from build123d import *

# Parameters (mm, degrees)
SKETCH1_W                    = 45.4
SKETCH1_H                    = 27
BOSS_EXTRUDE1_DEPTH          = 6
SKETCH4_W                    = 45.4
SKETCH4_H                    = 6
BOSS_EXTRUDE2_DEPTH          = 35
FILLET3_R                    = 10
F_3_0MM_DOWEL_HOLE1_D        = 3
BOSS_EXTRUDE3_DEPTH          = 6
FILLET4_R                    = 6
F_3_0_3_DIAMETER_HOLE1_D     = 3
F_3_0_3_DIAMETER_HOLE1_DEPTH = 6
F_3_0_3_DIAMETER_HOLE1_TIP   = 0.901290929
F_3_0_3_DIAMETER_HOLE2_D     = 3
F_3_0_3_DIAMETER_HOLE2_DEPTH = 6
F_3_0_3_DIAMETER_HOLE2_TIP   = 0.901290929


with BuildPart() as part:
    # Sketch1 → Boss-Extrude1 (new body)
    with BuildSketch(Plane(origin=(0, 0, 0), x_dir=(1, 0, 0), z_dir=(0, 1, 0))):
        with Locations((22.7, 13.5)):
            Rectangle(SKETCH1_W, SKETCH1_H)
    extrude(amount=BOSS_EXTRUDE1_DEPTH)

    # Sketch4 → Boss-Extrude2 (add)
    with BuildSketch(Plane(origin=(0, 6, 0), x_dir=(1, 0, 0), z_dir=(0, 1, 0))):
        with Locations((22.7, 13.5)):
            Rectangle(SKETCH4_W, SKETCH4_H)
    extrude(amount=BOSS_EXTRUDE2_DEPTH)

    # Fillet3
    fillet3_edges = [part.edges().sort_by_distance(p)[0] for p in [
        (22.7, 6, -10.5),
        (22.7, 6, -16.5),
    ]]
    fillet(fillet3_edges, radius=FILLET3_R)

    # Ø3.0mm Dowel Hole1 (through all)
    with Locations(Plane(origin=(0, 16, 0), x_dir=(1, 0, 0), z_dir=(0, 1, 0))):
        with Locations((12.7, 23.5), (32.7, 23.5), (32.7, 3.5), (12.7, 3.5)):
            Hole(F_3_0MM_DOWEL_HOLE1_D / 2)

    # Sketch5 → Boss-Extrude3 (add)
    with BuildSketch(Plane(origin=(0, 41, 0), x_dir=(1, 0, 0), z_dir=(0, 1, 0))):
        with BuildLine():
            Line((45.4, 33.5), (28.7, 33.5))
            ThreePointArc((28.7, 33.5), (22.7, 27.5), (16.7, 33.5))
            Line((16.7, 33.5), (0, 33.5))
            Line((0, 33.5), (0, -6.5))
            Line((0, -6.5), (16.7, -6.5))
            ThreePointArc((16.7, -6.5), (22.7, -0.5), (28.7, -6.5))
            Line((28.7, -6.5), (45.4, -6.5))
            Line((45.4, -6.5), (45.4, 33.5))
        make_face()
    extrude(amount=BOSS_EXTRUDE3_DEPTH)

    # Fillet4
    fillet4_edges = [part.edges().sort_by_distance(p)[0] for p in [
        (22.7, 41, -10.5),
        (22.7, 41, -16.5),
    ]]
    fillet(fillet4_edges, radius=FILLET4_R)

    # Ø3.0 (3) Diameter Hole1
    with Locations(Plane.XY.offset(6.5)):
        with Locations((6, 44), (39.4, 44)):
            Hole(F_3_0_3_DIAMETER_HOLE1_D / 2, depth=F_3_0_3_DIAMETER_HOLE1_DEPTH)
            with Locations((0, 0, -(F_3_0_3_DIAMETER_HOLE1_DEPTH + F_3_0_3_DIAMETER_HOLE1_TIP / 2))):  # 118° drill point
                Cone(0, F_3_0_3_DIAMETER_HOLE1_D / 2, F_3_0_3_DIAMETER_HOLE1_TIP, mode=Mode.SUBTRACT)

    # Ø3.0 (3) Diameter Hole2
    with Locations(Plane(origin=(0, 0, -33.5), x_dir=(-1, 0, 0), z_dir=(0, 0, -1))):
        with Locations((-39.4, 44), (-6, 44)):
            Hole(F_3_0_3_DIAMETER_HOLE2_D / 2, depth=F_3_0_3_DIAMETER_HOLE2_DEPTH)
            with Locations((0, 0, -(F_3_0_3_DIAMETER_HOLE2_DEPTH + F_3_0_3_DIAMETER_HOLE2_TIP / 2))):  # 118° drill point
                Cone(0, F_3_0_3_DIAMETER_HOLE2_D / 2, F_3_0_3_DIAMETER_HOLE2_TIP, mode=Mode.SUBTRACT)

    # Sketch12 → Ø3.0 (3) Diameter Hole3 (revolve, cut)
    with BuildSketch(Plane(origin=(45.4, 38, -13.5), x_dir=(0, 0, -1), z_dir=(0, 1, 0))):
        Polygon((0, 0), (0, 12.901290929), (1.5, 12), (1.5, 0), align=None)
    f_3_0_3_diameter_hole3 = revolve(axis=Axis((51.75, 38, -13.5), (-1, 0, 0)), mode=Mode.SUBTRACT)

    # Mirror1: Ø3.0 (3) Diameter Hole3 across plane
    add(f_3_0_3_diameter_hole3.mirror(Plane.ZY.offset(-22.7)), mode=Mode.SUBTRACT)


solid = part.part
Read the model definition and answer for the solid it produces. Units are mm, in the model's axes. A direction names the side the tool comes from. Coordinates: 2 decimals unless noted, no trailing zeros. Loops run counter-clockwise (first coordinate to the right, second up) from the corner with the lowest first, then second, coordinate; pieces in that order, holes last.
Q1. Consider probe 1 along Z at (x, y) = (32.7, 2.75); probe 2 along X at (y, z) = (1.5, -23.5); probe 3 along Y at (x, z) = (41.75, -13.5). Determine where each line is inside the solid, lowest interval first.
Q2. Which of the six approach directions +Z, -Z, +X, -X, +Y, -Y give full straight-line access (tool end or side, diameter ignored) to faces 1 (the face through (22, 3, 0)), 2 (the face through (23.02, 8.85, -19.51)), 3 (the face through (22, 25, -10.5)), 4 (the face through (5.675, 42.536, -30.458)), 5 (the face through (32.01, 3.49, -22.17))?
Q3. Each of these flat-tipped pins is pushed along its axis until it touches: pin 1 Ø6.5 at (x, y) = (27.5, 4.5) entering from +Z; pin 2 Ø2.5 at (x, z) = (32.7, -3.5) entering from -Y; pin 3 Ø2 at (x, y) = (9, 20.5) entering from +Z; pin 4 Ø1.5 at (x, z) = (32, -19) entering from -Y. Where does it stop, or does it pass through?
Q4. The part is cut by section C-C on z = -23.5. Write down the section's boundary in (x, y).
Q5. The part is cut by section B-B on x = 3. Write down the section's boundary in (y, z).
Q6. The mould has two halves that part along Z. Classify faces 6 (the face through (6.325, 42.536, 3.458)), 7 (the face through (5.916, 39.464, -13.175)), 8 (the face through (8, 44, -33.5)): +Z half, -Z half, draft (parallel to the pull), parting line (faces both ways), or undercut.
Q7. The part is cut by section A-A on z = -29.5. Write down the section's boundary in (x, y).
Q8. The part is cut by section D-D on x = 24. Write down the section's boundary in (y, z), and give its area (3 significant figures).
Results below:
1. probe 1: z = -27 to -25, -22 to -5, -2 to 0
1. probe 2: x = 0 to 11.2, 14.2 to 31.2, 34.2 to 45.4
1. probe 3: y = 0 to 36.5, 39.5 to 47
2. face 1: +Z, +X, -X, -Y
2. face 2: -Z, +X, -X
2. face 3: +Z, +X, -X
2. face 4: -Z
2. face 5: -Y
3. pin 1: stops at z = 0
3. pin 2: stops at y = 40.99
3. pin 3: stops at z = -10.5
3. pin 4: stops at y = 0
4. outline: (0, 0) - (11.2, 0) - (11.2, 6.46) - (0, 6.46) - close; (0, 41) - (45.4, 41) - (45.4, 47) - (0, 47) - close; (14.2, 0) - (31.2, 0) - (31.2, 6.46) - (14.2, 6.46) - close; (34.2, 0) - (45.4, 0) - (45.4, 6.46) - (34.2, 6.46) - close
5. outline: (0, -27) - (6, -27) - (6, -26.5) arc R10 cw to (16, -16.5) - (35, -16.5) arc R6 cw to (41, -22.5) - (41, -33.5) - (47, -33.5) - (47, 6.5) - (41, 6.5) - (41, -4.5) arc R6 cw to (35, -10.5) - (16, -10.5) arc R10 cw to (6, -0.5) - (6, 0) - (0, 0) - close; hole circle Ø3 at (38, -13.5)
6. face 6: draft
6. face 7: undercut
6. face 8: -Z half
7. outline: (0, 41) - (18.23, 41) - (18.23, 47) - (0, 47) - close; (27.17, 41) - (45.4, 41) - (45.4, 47) - (27.17, 47) - close; hole circle Ø3 at (6, 44); hole circle Ø3 at (39.4, 44)
8. outline: (0, -27) - (6, -27) - (6, -26.5) arc R10 cw to (16, -16.5) - (35, -16.5) arc R6 cw to (41, -22.5) - (41, -27.64) - (47, -27.64) - (47, 0.64) - (41, 0.64) - (41, -4.5) arc R6 cw to (35, -10.5) - (16, -10.5) arc R10 cw to (6, -0.5) - (6, 0) - (0, 0) - close
8. area: 600 mm2
